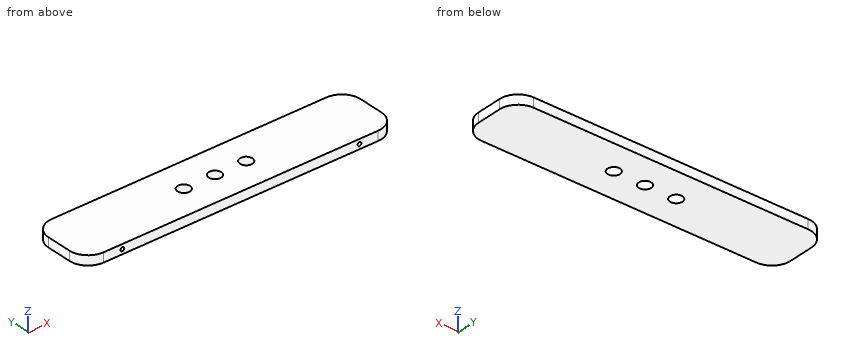
from build123d import *

# Parameters (mm, degrees)
BOSS_EXTRU_1_DEPTH      = 15
ESQUISSE2_R             = 10
ENL_V_MAT_EXTRU_2_DEPTH = 511.122534299
ESQUISSE3_R             = 3
ENL_V_MAT_EXTRU_3_DEPTH = 20


with BuildPart() as part:
    # Esquisse1 → Boss.-Extru.1 (new body)
    with BuildSketch(Plane.XY):
        with BuildLine():
            Line((30, 0), (470, 0))
            ThreePointArc((470, 0), (491.213203436, 8.786796564), (500, 30))
            Line((500, 30), (500, 70))
            ThreePointArc((500, 70), (491.213203436, 91.213203436), (470, 100))
            Line((470, 100), (30, 100))
            ThreePointArc((30, 100), (8.786796564, 91.213203436), (0, 70))
            Line((0, 70), (0, 30))
            ThreePointArc((0, 30), (8.786796564, 8.786796564), (30, 0))
        make_face()
    extrude(amount=BOSS_EXTRU_1_DEPTH)

    # Esquisse2 → Enlèv. mat.-Extru.2 (cut, through all)
    with BuildSketch(Plane.XY.offset(15)):
        with Locations((200, 50)):
            Circle(ESQUISSE2_R)
        with Locations((250, 50)):
            Circle(ESQUISSE2_R)
        with Locations((300, 50)):
            Circle(ESQUISSE2_R)
    extrude(amount=-ENL_V_MAT_EXTRU_2_DEPTH, mode=Mode.SUBTRACT)

    # Esquisse3 → Enlèv. mat.-Extru.3 (cut)
    with BuildSketch(Plane.XZ):
        with Locations(Location((60, 7.5, 0), (0, 0, 270))):
            Circle(ESQUISSE3_R)
        with Locations(Location((440, 7.5, 0), (0, 0, 270))):
            Circle(ESQUISSE3_R)
    extrude(amount=-ENL_V_MAT_EXTRU_3_DEPTH, mode=Mode.SUBTRACT)


solid = part.part
Design review of the part built by this model. Coordinates are the model's own, in mm. Give positions to 0.01 mm unless a question says otherwise; leave off trailing zeros. Order: outer loops, then holes, each group sorted by start corner. A loop starts at its lowest first (then second) coordinate and runs counter-clockwise, first axis right, second up. Notation, with made-up numbers: (-21, -3) - (16, -3) arc R12 cw to (16, 20) - close; hole circle Ø7 at (45.25, 76). An arc over 180 degrees is marked (long way). Use CSV: the item, a comma, the result in double quotes. Start each with the question number.
Q1. Take a section at C-C (y = 90.5). State the section outline as (x, z) points.
Q2. Take a section at A-A (z = 2.25). State the section outline as (x, y) points, and give its area (3 significant figures).
Q3. Take a section at B-B (x = 300). State the section outline as (y, z) points, and give its area (3 significant figures).
Q4. For line 1 (Z direction, x = 440, y = 10.25); line 2 (X direction, y = 14.75, z = 7.5); line 3 (X direction, y = 7.75, z = 7.5), list the stretches that pass through material, from the lowest coordinate up.
Calculated:
1,outline,"(8.1, 0) - (491.9, 0) - (491.9, 15) - (8.1, 15) - close"
2,outline,"(0, 30) arc R30 ccw to (30, 0) - (470, 0) arc R30 ccw to (500, 30) - (500, 70) arc R30 ccw to (470, 100) - (30, 100) arc R30 ccw to (0, 70) - close; hole circle Ø20 at (200, 50); hole circle Ø20 at (250, 50); hole circle Ø20 at (300, 50)"
2,area,"48,300 mm²"
3,outline,"(0, 0) - (40, 0) - (40, 15) - (0, 15) - close; (60, 0) - (100, 0) - (100, 15) - (60, 15) - close"
3,area,"1,200 mm²"
4,line 1,"z = 0 to 4.5, 10.5 to 15"
4,line 2,"x = 4.17 to 57, 63 to 437, 443 to 495.83"
4,line 3,"x = 9.88 to 57, 63 to 437, 443 to 490.12"
